The listing builds one solid part. Answer for the finished solid, in the listing's coordinates (mm). A direction names the side the tool comes from. Coordinates: 2 decimals unless noted, no trailing zeros. Loops run counter-clockwise (first coordinate to the right, second up) from the corner with the lowest first, then second, coordinate; pieces in that order, holes last. Notation, with made-up numbers: (64.5, -5.5) - (95.5, -5.5) arc R18 ccw to (95.5, 3.5) - close; hole circle Ø5 at (33, 66). An arc over 180 degrees is marked (long way). One line per question, with ' | ' between items.
from build123d import *

# Parameters (mm, degrees)
F0_R     = 3.5
F1_DEPTH = 2
F2_DEPTH = 23
F3_W     = 11.3556964174
F3_H     = 13.5
F4_DEPTH = 2
F5_DEPTH = 6


with BuildPart() as f1:
    # F0 (on Top) → F1 (new body)
    with BuildSketch(Plane.XY):
        Polygon((-4.6443035826, -6.75), (-4.6443035826, -4.75), (-10.3221517913, -4.75), (-16, -4.75), (-16, -6.75), align=None)
        with BuildLine():
            Line((-10.3221517913, -4.75), (-4.6443035826, -4.75))
            Line((-4.6443035826, -4.75), (-4.6443035826, 4.75))
            Line((-4.6443035826, 4.75), (-10.3221517821, 4.75))
            ThreePointArc((-10.3221517821, 4.75), (-6.9633945774, 3.3587572074), (-5.5721517913, 0))
            ThreePointArc((-5.5721517913, 0), (-6.9633945807, -3.3587572106), (-10.3221517913, -4.75))
        make_face()
        with BuildLine():
            Line((-16, -4.75), (-10.3221517913, -4.75))
            ThreePointArc((-10.3221517913, -4.75), (-15.0721517913, 4.6e-09), (-10.3221517821, 4.75))
            Line((-10.3221517821, 4.75), (-16, 4.75))
            Line((-16, 4.75), (-16, -4.75))
        make_face()
        with BuildLine():
            ThreePointArc((-10.3221517821, 4.75), (-15.0721517913, 4.6e-09), (-10.3221517913, -4.75))
            ThreePointArc((-10.3221517913, -4.75), (-6.9633945807, -3.3587572106), (-5.5721517913, 0))
            ThreePointArc((-5.5721517913, 0), (-6.9633945774, 3.3587572074), (-10.3221517821, 4.75))
        make_face()
        with Locations((-10.3221517913, 0)):
            Circle(F0_R, mode=Mode.SUBTRACT)
        Polygon((-10.3221517821, 4.75), (-4.6443035826, 4.75), (-4.6443035826, 6.75), (-16, 6.75), (-16, 4.75), align=None)
        with Locations((-10.3221517913, 0)):
            Circle(F0_R)
    extrude(amount=F1_DEPTH)

    # F0 (on Top) → F2 (join)
    with BuildSketch(Plane.XY):
        Polygon((-10.3221517821, 4.75), (-4.6443035826, 4.75), (-4.6443035826, 6.75), (-16, 6.75), (-16, 4.75), align=None)
        Polygon((-4.6443035826, -6.75), (-4.6443035826, -4.75), (-10.3221517913, -4.75), (-16, -4.75), (-16, -6.75), align=None)
    extrude(amount=F2_DEPTH)

    # F3 (on face) → F4 (join)
    with BuildSketch(Plane.XY.offset(23)):
        with Locations((-10.3221517913, 0)):
            Rectangle(F3_W, F3_H)
    extrude(amount=F4_DEPTH)

    # F0 (on Top) → F5 (join)
    with BuildSketch(Plane.XY):
        with BuildLine():
            ThreePointArc((-10.3221517821, 4.75), (-15.0721517913, 4.6e-09), (-10.3221517913, -4.75))
            ThreePointArc((-10.3221517913, -4.75), (-6.9633945807, -3.3587572106), (-5.5721517913, 0))
            ThreePointArc((-5.5721517913, 0), (-6.9633945774, 3.3587572074), (-10.3221517821, 4.75))
        make_face()
        with Locations((-10.3221517913, 0)):
            Circle(F0_R, mode=Mode.SUBTRACT)
    extrude(amount=-F5_DEPTH)


solid = f1.part
Item 1: The mould has two halves that part along Z. Classify faces 4 (the face through (-10, 0, 23)), 5 (the face through (-10, 0, 0)), 6 (the face through (-10, 6.75, 12)): pulls with the +Z half, pulls with the -Z half, needs draft (parallel to the pull), parting line crosses it, or undercut.
Taken from the geometry:
face 4: undercut | face 5: pulls with the -Z half | face 6: needs draft
Item 2: Find section B-B, the plane y = -1.5. Write down the section's boundary in (x, z).
Taken from the geometry:
outline: (-16, 0) - (-14.83, 0) - (-14.83, -6) - (-13.48, -6) - (-13.48, 0) - (-7.16, 0) - (-7.16, -6) - (-5.82, -6) - (-5.82, 0) - (-4.64, 0) - (-4.64, 2) - (-16, 2) - close; (-16, 23) - (-4.64, 23) - (-4.64, 25) - (-16, 25) - close
Item 3: Find the intervals of material crossed by line 1 (Z direction, x = -6.5, y = -1); line 2 (Z direction, x = -5.75, y = -3); line 3 (Y direction, x = -8, z = 9), in increasing order. Write a range as [from, to].
Taken from the geometry:
line 1: z = [-6, 2], [23, 25] | line 2: z = [0, 2], [23, 25] | line 3: y = [-6.75, -4.75], [4.75, 6.75]
Item 4: This flat-tipped pin is pushed along its axis until it touches: pin 1 Ø2 at (x, y) = (-10.5, -1.5) entering from -Z. Where does it stop, or does it pass through?
Taken from the geometry:
pin 1: stops at z = 0
Item 5: Find section C-C, the plane x = -10.75. Write down the section's boundary in (y, z).
Taken from the geometry:
outline: (-6.75, 0) - (-4.73, 0) - (-4.73, -6) - (-3.47, -6) - (-3.47, 0) - (3.47, 0) - (3.47, -6) - (4.73, -6) - (4.73, 0) - (6.75, 0) - (6.75, 25) - (-6.75, 25) - close; hole (-4.75, 2) - (4.75, 2) - (4.75, 23) - (-4.75, 23) - close
Item 6: Which of the six approach directions +Z, -Z, +X, -X, +Y, -Y give full straight-line access (tool end or side, diameter ignored) to faces 1 (the face through (-10, 0, 2)), 2 (the face through (-7, 1.1, -3)), 3 (the face through (-16, 6, 12))?
Taken from the geometry:
face 1: +X, -X | face 2: -Z | face 3: +Z, -Z, -X, +Y, -Y
Item 7: Find section D-D, the plane z = -2. Write down the section's boundary in (x, y), plus the area to 3 significant figures.
Taken from the geometry:
outline: circle Ø9.5 at (-10.32, 0); hole circle Ø7 at (-10.32, 0) | area: 32.4 mm2
Item 8: Find section A-A, the plane z = 12.5. Write down the section's boundary in (x, y), plus the area to 3 significant figures.
Taken from the geometry:
outline: (-16, -6.75) - (-4.64, -6.75) - (-4.64, -4.75) - (-16, -4.75) - close; (-16, 4.75) - (-4.64, 4.75) - (-4.64, 6.75) - (-16, 6.75) - close | area: 45.4 mm2
